Model file for the job. Use its own axes, mm. Face numbers are marked on the shaded views. A direction names the side the tool comes from. Round coordinates to 2 decimals unless told otherwise and drop trailing zeros. Write each loop counter-clockwise with the first axis right and the second up, starting at its lowest first coordinate (ties: lowest second). Pieces come first, ordered by that corner, then holes. Notation, with made-up numbers: (5.25, -18.5) - (60.25, -18.5) arc R21 cw to (60.25, 17.5) - close; hole circle Ø6 at (12, -39.5). An arc over 180 degrees is marked (long way). One line per item, written item: value.
Autodesk Inventor part; units mm, degrees
ref_plane "Work Plane1" through (0, 0, 2.5) normal (0, 0, -1) x (-1, 0, 0)
ref_plane "Work Plane3" through (-100, -40, 5) normal (0, -1, 0) x (1, 0, 0)
ref_plane "Work Plane5" through (-100, -50, 5) normal (0, -1, 0) x (1, 0, 0)
sketch "Sketch1" plane through (0, 0, 0) normal (0, 0, 1) x (1, 0, 0)
  line L0 (-110, 50) -> (110, 50)
  line L1 (110, 50) -> (110, -50)
  line L2 (110, -50) -> (-110, -50)
  line L3 (-110, -50) -> (-110, 50)
  line L4 (-110, 50) -> (110, -50) construction
  line L5 (110, 50) -> (-110, -50) construction
  line L6 (110, 50) -> (100, 50)
  line L7 (100, 50) -> (100, -50)
  line L8 (100, -50) -> (110, -50)
  line L9 (110, -50) -> (110, 50)
  line L10 (-110, 50) -> (-100, 50)
  line L11 (-100, 50) -> (-100, -50)
  line L12 (-100, -50) -> (-110, -50)
  line L13 (-110, -50) -> (-110, 50)
  point P0 (0, 0)
  dimension "d0" = 220
  dimension "d1" = 100
  dimension "d2" = 10
  dimension "d3" = 10
extrude "Extrusion1" add sketch "Sketch1" along normal blind 5 contours L0 L7 L2 L11
extrude "Extrusion2" add sketch "Sketch1" along normal blind 30 contours L0 L11 L2 L3 | L0 L1 L2 L7
sketch "Sketch2" plane through (110, -50, 0) normal (1, 0, 0) x (0, 0, -1)
  circle A0 centre (-15, 75) radius 1.5
  circle A1 centre (-15, 25) radius 1.5
  line L0 (0, 100) -> (-30, 100)
  line L1 (0, 0) -> (-30, 0)
  point P0 (0, 50)
  point P1 (-15, 100)
  point P2 (-15, 0)
  dimension "d8" = 3
  dimension "d9" = 3
  dimension "d10" = 25
  dimension "d11" = 25
extrude "Extrusion3" cut sketch "Sketch2" against normal blind 300
ref_plane "Work Plane1" through (0, 0, 2.5) normal (0, 0, -1) x (-1, 0, 0)
sketch "Sketch5" plane through (-100, -50, 5) normal (0, -1, 0) x (1, 0, 0)
  point P0 (100, -5)
sketch "Sketch6" plane through (0, 0, 0) normal (0, 0, -1) x (-1, 0, 0)
  line L0 (-110, 50) -> (110, 50)
  line L1 (-90, 50) -> (-75, 50)
  point P0 (0, 0)
sketch "Sketch7" plane through (-100, -50, 5) normal (0, -1, 0) x (1, 0, 0)
  point P0 (100, -5)
sketch "Sketch10" plane through (0, 0, 0) normal (0, 0, -1) x (-1, 0, 0)
  point P0 (0, 0)
sketch "Sketch11" plane through (-100, -50, 5) normal (0, -1, 0) x (1, 0, 0)
  point P0 (100, -5)
sketch "Sketch12" plane through (-100, -50, 5) normal (0, -1, 0) x (1, 0, 0)
  point P0 (100, -5)
sketch "Sketch13" plane through (-100, -50, 5) normal (0, -1, 0) x (1, 0, 0)
  point P0 (100, -5)
sketch "Sketch14" plane through (-100, -50, 5) normal (0, -1, 0) x (1, 0, 0)
  point P0 (100, -5)
ref_plane "Work Plane3" through (-100, -40, 5) normal (0, -1, 0) x (1, 0, 0)
sketch "Sketch16" plane through (0, 0, 0) normal (0, 0, -1) x (-1, 0, 0)
  point P0 (0, 0)
sketch "Sketch18" plane through (-100, -50, 5) normal (0, -1, 0) x (1, 0, 0)
  point P0 (100, -5)
sketch "Sketch20" plane through (0, 0, 0) normal (0, 0, -1) x (-1, 0, 0)
  line L0 (-110, 50) -> (110, 50)
  line L1 (100, -50) -> (-100, -50)
  line L2 (-110, 50) -> (-90, 50)
  line L3 (-90, 50) -> (-90, -50)
  line L4 (-90, -50) -> (-110, -50)
  line L5 (-110, -50) -> (-110, 50)
  line L6 (-100, 50) -> (100, 50)
  line L7 (-74.75, 50) -> (-54.75, 50)
  line L8 (-54.75, 50) -> (-54.75, -50)
  line L9 (-54.75, -50) -> (-74.75, -50)
  line L10 (-74.75, -50) -> (-74.75, 50)
  point P0 (0, 0)
  point P1 (-74.75, 50)
  point P2 (-74.75, -50)
  dimension "d46" = 20
  dimension "d47" = 20
  dimension "d48" = 15.25
extrude "Extrusion10" add sketch "Sketch20" along normal blind 15 contours L0 L3 L1 L4 L5 | L0 L8 L1 L10
ref_plane "Work Plane5" through (-100, -50, 5) normal (0, -1, 0) x (1, 0, 0)
sketch "Sketch22" plane through (-100, -50, 5) normal (0, -1, 0) x (1, 0, 0)
  line L0 (174.75, -5) -> (190, -5)
  line L1 (182.375, -5) -> (182.375, -19.781)
  arc A0 (174.1976, -13.8453) -> (174.1552, -16.1739) centre (172.7726, -14.984) ccw
  arc A1 (174.184, -13.8286) -> (174.1552, -16.1739) centre (172.7726, -14.984) ccw
  arc A2 (174.184, -13.8286) -> (174.5946, -13.637) centre (174.3446, -13.637) ccw
  line L2 (174.5946, -13.637) -> (174.5946, -4.5959)
  line L3 (174.5946, -4.5959) -> (190.095, -4.5959)
  line L4 (190.095, -4.5959) -> (190.095, -13.6504)
  arc A3 (190.095, -13.6504) -> (190.5052, -13.8286) centre (190.3446, -13.637) ccw
  arc A4 (190.5341, -16.1739) -> (190.5052, -13.8286) centre (191.9167, -14.984) ccw
  arc A5 (190.5341, -16.1739) -> (190.0946, -16.337) centre (190.3446, -16.337) ccw
  line L5 (190.0946, -16.337) -> (190.0946, -19.8904)
  line L6 (190.0946, -19.8904) -> (174.5946, -19.8904)
  line L7 (174.5946, -19.8904) -> (174.5946, -16.337)
  arc A6 (174.5946, -16.337) -> (174.1552, -16.1739) centre (174.3446, -16.337) ccw
  line L8 (174.75, -5) -> (174.75, -20)
  circle A7 centre (182.375, -12.3905) radius 0.9755 construction
  line L9 (190, -5) -> (190, -20)
  line L10 (154.75, -5) -> (154.75, -20)
  line L11 (174.75, -20) -> (154.75, -20)
  line L12 (154.75, -20) -> (154.75, -18)
  line L13 (154.75, -18) -> (174.75, -18)
  line L14 (174.75, -18) -> (174.75, -20)
  point P0 (100, -5)
  point P1 (182.7765, -10.9918)
  point P2 (174.184, -13.8286)
  point P3 (174.75, -19.8904)
  point P4 (190, -19.8904)
  point P5 (174.5946, -18)
  dimension "d74" = 2
extrude "Extrusion13" cut sketch "Sketch22" against normal blind 95 contours L8 L13 L7 A6 A0 A2 L2 L3 L4 A3 A4 A5 L5 L6 L9 L0 | L8 L6 L7 L13
sketch "Sketch23" plane through (0, 0, 0) normal (0, 0, -1) x (-1, 0, 0)
  line L0 (110, -50) -> (-54.75, -50)
  line L1 (-54.75, 50) -> (-54.75, -50)
  line L2 (110, -50) -> (-54.75, -50)
  line L3 (-54.75, -50) -> (-54.75, 50)
  line L4 (-54.75, 50) -> (110, 50)
  line L5 (110, 50) -> (110, -50)
  point P0 (0, 0)
extrude "Extrusion14" add sketch "Sketch23" along normal blind 10
extrude "Extrusion15" cut sketch "Sketch22" against normal blind 100 contours L8 L11 L10 L13 L7 L6
sketch "Sketch24" plane through (110, -50, 30) normal (1, 0, 0) x (0, 0, -1)
  line L0 (45, 100) -> (0, 100)
  line L1 (45, 100) -> (33.2, 100)
  line L2 (33.2, 100) -> (33.2, 50)
  line L3 (33.2, 50) -> (45, 50)
  line L4 (45, 50) -> (45, 100)
  point P0 (30, 50)
  dimension "d77" = 11.8
extrude "Extrusion16" cut sketch "Sketch24" against normal blind 9
sketch "Sketch25" plane through (110, -50, 30) normal (1, 0, 0) x (0, 0, -1)
  line L0 (40, 100) -> (0, 100)
  line L1 (33.2, 100) -> (23.2, 100)
  line L2 (23.2, 100) -> (23.2, 50)
  line L3 (23.2, 50) -> (33.2, 50)
  line L4 (33.2, 50) -> (33.2, 100)
  line L5 (33.2, 50) -> (33.2, 100)
  point P0 (30, 50)
  dimension "d80" = 10
extrude "Extrusion17" add sketch "Sketch25" along normal blind 45
sketch "Sketch26" plane through (110, 0, 6.8) normal (0, 0, 1) x (1, 0, 0)
  line L0 (0, 0) -> (0, 50)
  line L1 (0, 0) -> (45, 0)
  line L2 (45, 50) -> (45, 0)
  line L3 (0, 50) -> (45, 50)
  point P0 (-110, 0)
extrude "Extrusion18" cut sketch "Sketch26" against normal blind 4
properties part number "offloadbase"
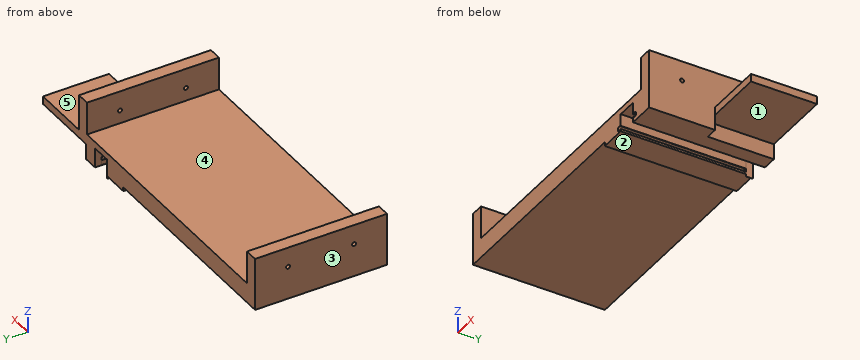
1. Band-saw the part on A-A on z = 7.5. Write the cut outline in (x, y), plus the area to 3 significant figures.
Report:
outline: (-110, -50) - (-100, -50) - (-100, 50) - (-110, 50) - close; (100, -50) - (110, -50) - (110, 50) - (100, 50) - close
area: 2,000 mm²
2. Wall check: probe 1 along Y at (x, z) = (107, 15); probe 2 along X at (y, z) = (-43.5, 9.5); probe 3 along X at (y, z) = (-40.5, -12). Give the ranges that are in metal, low to high. Write a range as [from, to].
Report:
probe 1: [-50, -26.5], [-23.5, 23.5], [26.5, 50]
probe 2: [-110, -100], [100, 110]
probe 3: [54.75, 74.59], [90.09, 110]
3. Drop flat-ended pins along their axis: pin 1 (3 mm diameter, centred on x = 33.5, y = -37.5, fed in from -Z); pin 2 (3.5 mm diameter, centred on y = -25, z = 15, fed in from +X); pin 3 (0.6 mm diameter, centred on y = 47.5, z = -14, fed in from -X). Give the stop position or say it passes through.
Report:
pin 1: z = -10
pin 2: x = 110
pin 3: x = 74.59
4. Band-saw the part on D-D on x = 137. Write the cut outline in (y, z), plus the area to 3 significant figures.
Report:
outline: (0, -3.2) - (50, -3.2) - (50, 2.8) - (0, 2.8) - close
area: 300 mm²
5. Band-saw the part on C-C on y = -2.5. Write the cut outline in (x, z) (3 decimals).
Report:
outline: (-110, -10) - (54.75, -10) - (54.75, -13) - (74.595, -13) - (74.595, -11.337) arc R0.25 ccw to (74.155, -11.174) arc R1.824 cw (long way) to (74.184, -8.829) arc R0.25 ccw to (74.595, -8.637) - (74.595, 0.404) - (90.095, 0.404) - (90.095, -8.65) arc R0.25 ccw to (90.505, -8.829) arc R1.824 cw (long way) to (90.534, -11.174) arc R0.25 ccw to (90.095, -11.337) - (90.095, -14.89) - (90, -14.89) - (90, -15) - (110, -15) - (110, 30) - (100, 30) - (100, 5) - (-100, 5) - (-100, 30) - (-110, 30) - close
6. Band-saw the part on B-B on x = -53. Write the cut outline in (y, z).
Report:
outline: (-50, -10) - (50, -10) - (50, 5) - (-50, 5) - close
7. Tool access for the marked faces 1, 2, 3, 4 and 5: list every direction of +Z, -Z, +X, -X, +Y, -Y with a clear straight run to the whole face (end or side of a thin tool).
Report:
face 1: -Z, +X, +Y
face 2: -Z, -X, +Y, -Y
face 3: +Z, -Z, -X, +Y, -Y
face 4: +Z, +Y, -Y
face 5: +Z, +X, +Y, -Y
